Autodesk Inventor part; units mm, degrees
ref_plane "YZ Plane" through (0, 0, 0) normal (1, 0, 0) x (0, 1, 0)
ref_plane "XZ Plane" through (0, 0, 0) normal (0, 1, 0) x (-1, 0, 0)
ref_plane "XY Plane" through (0, 0, 0) normal (0, 0, 1) x (1, 0, 0)
sketch "Sketch1" plane through (0, 0, 0) normal (0, 1, 0) x (-1, 0, 0)
  circle A0 centre (0, 0) radius 2.5
  circle A1 centre (0, 0) radius 1.6
  line L0 (4, -4) -> (-4, -4)
  line L1 (-4, -4) -> (-4, 4)
  line L2 (-4, 4) -> (4, 4)
  line L3 (4, 4) -> (4, -4)
  line L4 (4, -4) -> (-4, 4) construction
  line L5 (-4, -4) -> (4, 4) construction
  dimension "d0" = 5
  dimension "d1" = 3.2
  dimension "d11" = 8
  dimension "d12" = 8
extrude "Extrusion1" add sketch "Sketch1" along normal blind 8 contours A0 | L0 L1 L2 L3
fillet "Fillet1" radius 2 4 edges at (4, 4, 4) (-4, 4, 4) (4, 4, -4) (-4, 4, -4)
properties part number "8mm Spacer"
Work out the finished part from the listing and answer in its coordinate system (mm). Give positions to 0.01 mm unless a question says otherwise; leave off trailing zeros. Write each loop counter-clockwise with the first axis right and the second up, starting at its lowest first coordinate (ties: lowest second). Pieces come first, ordered by that corner, then holes. Notation, with made-up numbers: (36.25, -10) -> (69.25, -10) arc R12 ccw to (69.25, 1) -> close; hole circle Ø6 at (-28, 31). An arc over 180 degrees is marked (long way). Write item = value, one per line.
Q1. Section D-D on z = -3.25 is taken. Determine the outline of the cut face in (x, y).
Computed values:
outline = (-3.56, 0) -> (3.56, 0) -> (3.56, 8) -> (-3.56, 8) -> close
Q2. Flat-ended cylindrical pins translate along their axes: pin 1 Ø1.5 at (y, z) = (7, 3) entering from +X; pin 2 Ø2.5 at (x, z) = (0, 0) entering from -Y; pin 3 Ø3 at (x, y) = (-3, 3.5) entering from -Z. Find the tip coordinate at first contact, or state that the pin passes through.
Computed values:
pin_1 = 3.98
pin_2 = through
pin_3 = -4
Q3. Consider line 1 along Z through (x, y) = (0, 5); line 2 along X through (y, z) = (7.5, 0.25); line 3 along X through (y, z) = (4.25, 3.5). Determine where each line is inside the solid, lowest interval first.
Computed values:
line_1 = -4 to -1.6, 1.6 to 4
line_2 = -4 to -1.58, 1.58 to 4
line_3 = -3.32 to 3.32
Q4. Section B-B on x = 0 is taken. Determine the outline of the cut face in (y, z).
Computed values:
outline = (0, -4) -> (8, -4) -> (8, -1.6) -> (0, -1.6) -> close; (0, 1.6) -> (8, 1.6) -> (8, 4) -> (0, 4) -> close
Q5. Section A-A on z = 0 is taken. Determine the outline of the cut face in (x, y).
Computed values:
outline = (-4, 0) -> (-1.6, 0) -> (-1.6, 8) -> (-4, 8) -> close; (1.6, 0) -> (4, 0) -> (4, 8) -> (1.6, 8) -> close
Q6. Section C-C on y = 3.5 is taken. Determine the outline of the cut face in (x, z), and give its area (3 significant figures).
Computed values:
outline = (-4, -2) arc R2 ccw to (-2, -4) -> (2, -4) arc R2 ccw to (4, -2) -> (4, 2) arc R2 ccw to (2, 4) -> (-2, 4) arc R2 ccw to (-4, 2) -> close; hole circle Ø3.2 at (0, 0)
area = 52.5 mm^2
Q7. For a pull along X with two mould halves and no side action, classify faces 1 (the cylindrical face through (3.43, 4.06, -3.4)), 2 (the cylindrical face through (-3.4, 4.06, -3.43)), 3 (the cylindrical face through (1.27, 3.94, 0.97)), 4 (the flat face through (0, 4, 4)) as pulls with the +X half, pulls with the -X half, needs draft (parallel to the pull), parting line crosses it, or undercut.
Computed values:
face_1 = pulls with the +X half
face_2 = pulls with the -X half
face_3 = undercut
face_4 = needs draft
